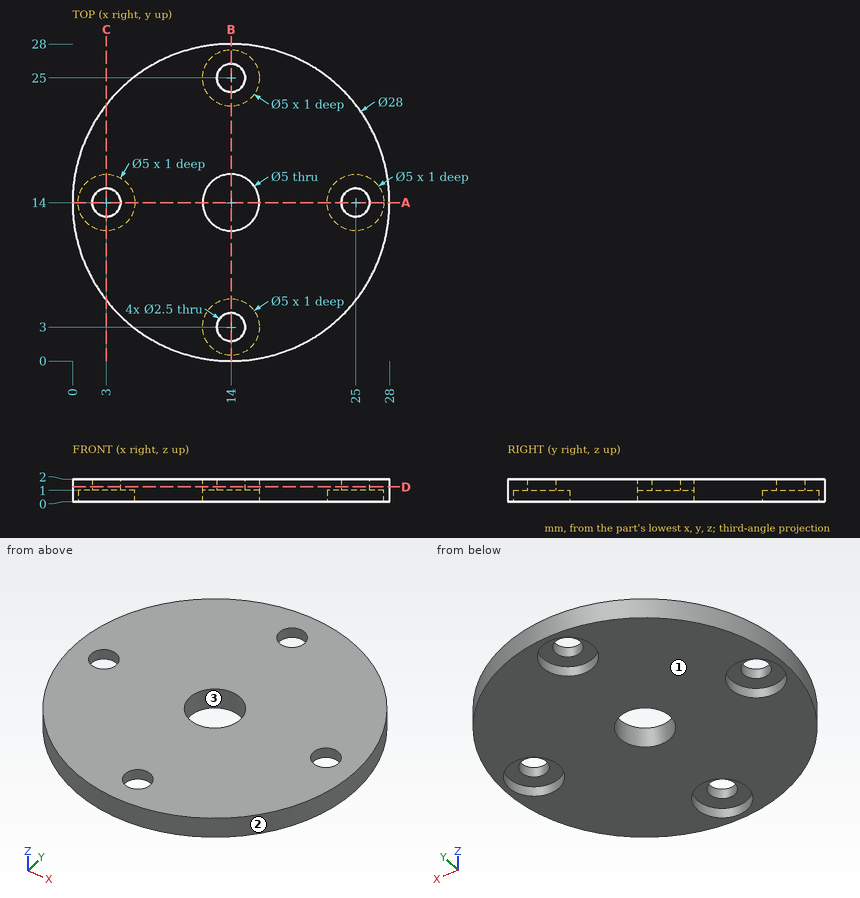
Print and shaded views of the part. All mm, measured from the part's lowest x, y and z. Round coordinates to 2 decimals unless told otherwise and drop trailing zeros. Write each loop counter-clockwise with the first axis right and the second up, starting at its lowest first coordinate (ties: lowest second). Pieces come first, ordered by that corner, then holes. Notation, with made-up numbers: (52.5, 77) - (64.5, 77) arc R24 cw to (64.5, 92) - close; hole circle Ø11 at (-29, 51). An arc over 180 degrees is marked (long way). Write each question's results on one line, items separated by ' | '. Start each with the question number.
Item 1: Drop a flat-ended pin along its axis: P1, Ø1.5, axis at x = 13, y = 3, coming from the -Z side. Give the stop position or say it passes through.
Item 2: Saw through at A-A (y = 14). Write the cut outline in (x, z), and give its area (3 significant figures).
Item 3: Saw through at D-D (z = 1.3). Write the cut outline in (x, y), and give its area (3 significant figures).
Item 4: Saw through at C-C (x = 3). Write the cut outline in (y, z).
Item 5: Mould opens along X. For the marked faces 1, 2 and 3 say: pulls with the +X half, pulls with the -X half, needs draft (parallel to the pull), parting line crosses it, or undercut.
Item 6: Wall check: L1, parallel to Y at x = 14, z = 0.3; L2, parallel to Z at x = 16, y = 2; L3, parallel to X at y = 13.25, z = 1.3. Give the ranges that are in metal, low to high. Write a range as [from, to].
Results are:
1) P1: stops at z = 1
2) outline: (0, 0) - (0.5, 0) - (0.5, 1) - (1.75, 1) - (1.75, 2) - (0, 2) - close; (4.25, 1) - (5.5, 1) - (5.5, 0) - (11.5, 0) - (11.5, 2) - (4.25, 2) - close; (16.5, 0) - (22.5, 0) - (22.5, 1) - (23.75, 1) - (23.75, 2) - (16.5, 2) - close; (26.25, 1) - (27.5, 1) - (27.5, 0) - (28, 0) - (28, 2) - (26.25, 2) - close | area: 31.0 mm²
3) outline: circle Ø28 at (14, 14); hole circle Ø2.5 at (3, 14); hole circle Ø5 at (14, 14); hole circle Ø2.5 at (14, 3); hole circle Ø2.5 at (14, 25); hole circle Ø2.5 at (25, 14) | area: 576 mm²
4) outline: (5.34, 0) - (11.5, 0) - (11.5, 1) - (12.75, 1) - (12.75, 2) - (5.34, 2) - close; (15.25, 1) - (16.5, 1) - (16.5, 0) - (22.66, 0) - (22.66, 2) - (15.25, 2) - close
5) face 1: needs draft | face 2: parting line crosses it | face 3: undercut
6) L1: y = [0, 0.5], [5.5, 11.5], [16.5, 22.5], [27.5, 28] | L2: z = [1, 2] | L3: x = [0.02, 2], [4, 11.62], [16.38, 24], [26, 27.98]
